Can you work these out from the model? Positions are in its coordinate system, mm. Give positions to 0.01 mm unless a question says otherwise; leave off trailing zeros. Order: outer loops, then holes, each group sorted by start corner. A loop starts at its lowest first (then second) coordinate and runs counter-clockwise, first axis right, second up. Notation, with made-up numbers: (74.5, -25.5) - (117.5, -25.5) arc R20 cw to (117.5, 13.5) - close; hole circle Ø8 at (-28, 63.25). An arc over 180 degrees is marked (long way). Use one line per item in the form item = value. Start each with the question number.
1) Please list where these lines run through material, in increasing order: probe 1 along Y at (x, z) = (1, -0.2); probe 2 along Y at (x, z) = (28, -0.6).
2) Suppose I cut it at A-A, the plane x = -15.5. Write out the boundary of the cut face in (y, z), and give its area (3 significant figures).
3) For pin 1 (1 mm diameter, centred on x = 6, y = 0.5, fed in from -Z), with a flat end and sliding along its axis, tell me the tip position at first contact or that it passes through.
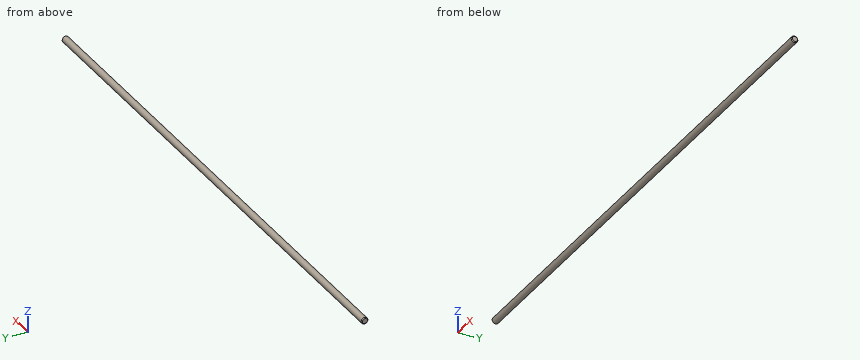
```python
from build123d import *

# Parameters (mm, degrees)
SKETCH2_R                = 1
BOSS_EXTRUDE1_DEPTH      = 82.175
BOSS_EXTRUDE1_DEPTH_BACK = 82.175
SKETCH5_OUTSIDE_W        = 367.574
SKETCH5_OUTSIDE_H        = 367.574
SKETCH5_OUTSIDE_R        = 0.75256417
CUT_EXTRUDE1_DEPTH       = 165.35
CUT_EXTRUDE1_TAPER       = 45


with BuildPart() as part:
    # Sketch2 → Boss-Extrude1 (new body, two sides)
    with BuildSketch(Plane(origin=(0, 0, 0), x_dir=(0, 0, -1), z_dir=(1, 0, 0))) as boss_extrude1_sk:
        Circle(SKETCH2_R)
    extrude(amount=BOSS_EXTRUDE1_DEPTH)
    extrude(boss_extrude1_sk.sketch, amount=-BOSS_EXTRUDE1_DEPTH_BACK)

    # Sketch5 outside → Cut-Extrude1 (cut, through all)
    with BuildSketch(Plane(origin=(82.175, 0, 0), x_dir=(0, 0, -1), z_dir=(1, 0, 0))):
        Rectangle(SKETCH5_OUTSIDE_W, SKETCH5_OUTSIDE_H)
        Circle(SKETCH5_OUTSIDE_R, mode=Mode.SUBTRACT)
    cut_extrude1 = extrude(amount=-CUT_EXTRUDE1_DEPTH, taper=CUT_EXTRUDE1_TAPER, mode=Mode.SUBTRACT)

    # Mirror1: Cut-Extrude1 across plane
    add(cut_extrude1.mirror(Plane(origin=(0, 0, 0), x_dir=(0, 0, 1), z_dir=(1, 0, 0))), mode=Mode.SUBTRACT)


solid = part.part
```
Result sheet:
q1.probe_1 = -0.98 to 0.98
q1.probe_2 = -0.8 to 0.8
q2.outline = circle Ø2 at (0, 0)
q2.area = 3.14 mm²
q3.pin_1 = -1
